Check sheet for the modelled part. Datum: model origin and axes. Units: mm. A direction names the side the tool comes from. Give positions to 0.01 mm unless a question says otherwise; leave off trailing zeros. Write each loop counter-clockwise with the first axis right and the second up, starting at its lowest first coordinate (ties: lowest second). Pieces come first, ordered by that corner, then holes. Notation, with made-up numbers: (86, -20) -> (129, -20) arc R25 cw to (129, 9) -> close; hole circle Ø9 at (40, 79.5). An arc over 180 degrees is marked (long way). Answer as a JSON object with one key per item and string values.
from build123d import *

# Parameters (mm, degrees)
BOSS_EXTRUDE1_DEPTH = 220
SHELL1_T            = -7


with BuildPart() as part:
    # Sketch1 → Boss-Extrude1 (new body)
    with BuildSketch(Plane(origin=(0, 0, 0), x_dir=(1, 0, 0), z_dir=(0, 1, 0))):
        with BuildLine():
            Line((-275, -200), (275, -200))
            ThreePointArc((275, -200), (292.67766953, -192.67766953), (300, -175))
            Line((300, -175), (300, 175))
            ThreePointArc((300, 175), (292.67766953, 192.67766953), (275, 200))
            Line((275, 200), (-275, 200))
            ThreePointArc((-275, 200), (-292.67766953, 192.67766953), (-300, 175))
            Line((-300, 175), (-300, -175))
            ThreePointArc((-300, -175), (-292.67766953, -192.67766953), (-275, -200))
        make_face()
    extrude(amount=BOSS_EXTRUDE1_DEPTH)

    # Shell1
    shell1_openings = [part.faces().sort_by_distance(p)[0] for p in [
        (0, 220, 0),
    ]]
    offset(amount=SHELL1_T, openings=shell1_openings, kind=Kind.INTERSECTION)


solid = part.part
1. Access from +Z, -Z, +X, -X, +Y, -Y to the whole of each face (thin tool, end or side, straight path). Record for faces 1 (the face through (287.867, 112.009, -187.587)), 2 (the face through (292.871, 108.46, -192.482)).
Determined:
{"face 1": "+Y", "face 2": "-Z, +X, +Y, -Y"}
2. Sectioned sample at C-C, the plane x = -147. Enter the section's corners in (y, z), plus the area to 3 significant figures.
Determined:
{"outline": "(0, -200) -> (220, -200) -> (220, -193) -> (7, -193) -> (7, 193) -> (220, 193) -> (220, 200) -> (0, 200) -> close", "area": "5,780 mm^2"}
3. Sectioned sample at A-A, the plane z = -125.5. Enter the section's corners in (x, y).
Determined:
{"outline": "(-300, 0) -> (300, 0) -> (300, 220) -> (293, 220) -> (293, 7) -> (-293, 7) -> (-293, 220) -> (-300, 220) -> close"}
4. Go/stop test with a flat-tipped pin: P1, Ø3, axis at x = 108.5, z = -50.5, coming from the +Y side. Record where the tip stops, or that it passes through.
Determined:
{"P1": "y = 7"}
5. Scan lines: L1, parallel to Z at x = -93.5, y = 171; L2, parallel to X at y = 18, z = 141.5; L3, parallel to Y at x = 198, z = -76. Record each from-to range of solid material in increasing order. Write a range as [from, to].
Determined:
{"L1": "[-200, -193], [193, 200]", "L2": "[-300, -293], [293, 300]", "L3": "[0, 7]"}
6. Sectioned sample at B-B, the plane y = 56.5. Enter the section's corners in (x, z), plus the area to 3 significant figures.
Determined:
{"outline": "(-300, -175) arc R25 ccw to (-275, -200) -> (275, -200) arc R25 ccw to (300, -175) -> (300, 175) arc R25 ccw to (275, 200) -> (-275, 200) arc R25 ccw to (-300, 175) -> close; hole (-293, -175) arc R18 ccw to (-275, -193) -> (275, -193) arc R18 ccw to (293, -175) -> (293, 175) arc R18 ccw to (275, 193) -> (-275, 193) arc R18 ccw to (-293, 175) -> close", "area": "13,500 mm^2"}
7. Mould release check, pull along Z, two halves, no side actions. Record for faces 3 (the face through (4, 108, -200)), 4 (the face through (-4, 0, -3)), 5 (the face through (293, 112, 2)): released by +Z, released by -Z, zero draft, split by the parting line, or undercut.
Determined:
{"face 3": "released by -Z", "face 4": "zero draft", "face 5": "undercut"}
